Design review of the part shown in the three views and the two pictorial views. Dimensions are in mm from the part's minimum x, y and z. A direction names the side the tool comes from. Give positions to 0.01 mm unless a question says otherwise; leave off trailing zeros. Write each loop counter-clockwise with the first axis right and the second up, starting at its lowest first coordinate (ties: lowest second). Pieces come first, ordered by that corner, then holes. Notation, with made-up numbers: (24.5, -35.5) -> (36.5, -35.5) arc R16 cw to (36.5, -11.5) -> close; hole circle Ø6 at (29, 20). An arc over 180 degrees is marked (long way). Return JSON: item names as keys, results as strings. Group by question number.
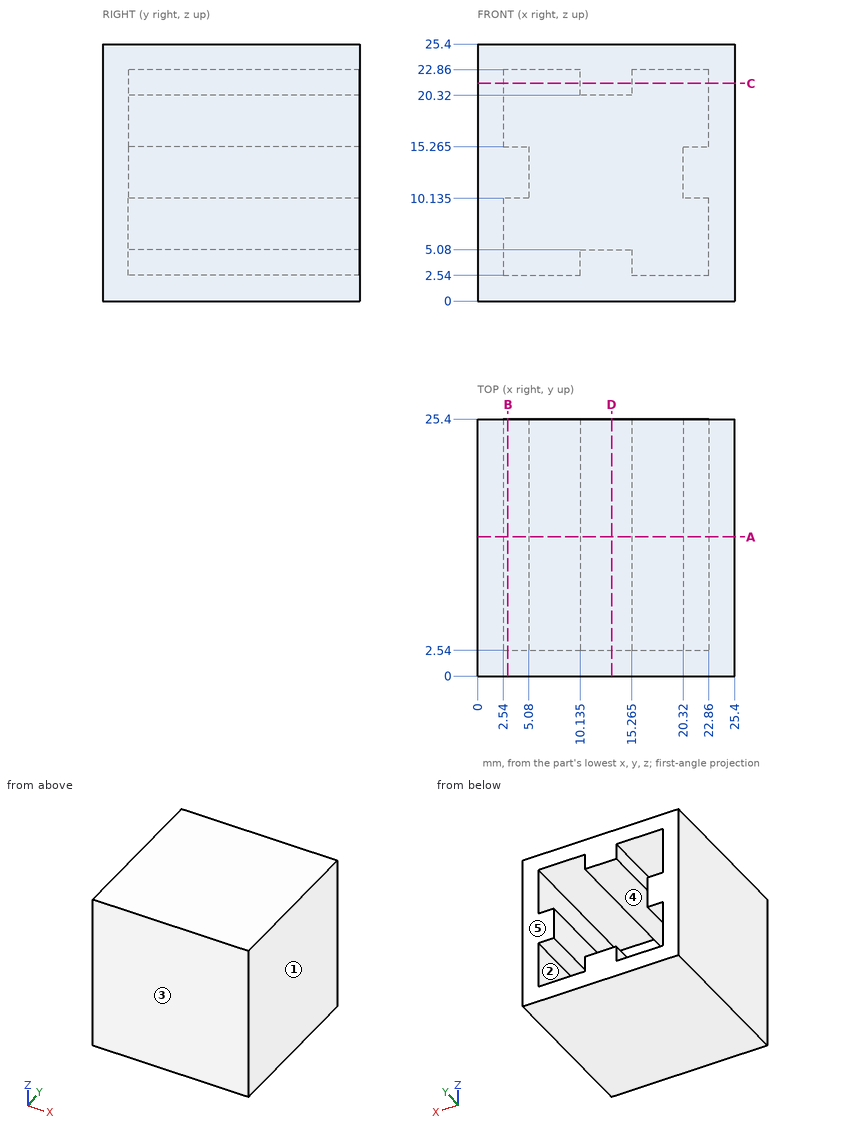
Q1. Take a section at B-B, the plane x = 3. Give the boundary of the cut face in (y, z) (3 decimals).
Q2. Take a section at C-C, the plane z = 21.5. Give the boundary of the cut face in (x, y) (3 decimals).
Q3. Tool access review of the marked faces 4 and 5: name each direction out of +Z, -Z, +X, -X, +Y, -Y from which nothing blocks a thin tool from reaching the whole face with its end or side.
Q4. For L1, parallel to X at y = 8, z = 3.5 (3 decimals); L2, parallel to X at y = 7.75, z = 8, list the stretches that pass through material, from the lowest coordinate up. Write a range as from..to.
Q5. Mouldability with a two-part tool opening along X and no side actions: class the marked faces 1, 2 and 3 as +X half, -X half, draft (parallel to the pull), parting line (faces both ways), or undercut.
Q6. Take a section at A-A, the plane y = 13.75. Give the boundary of the cut face in (x, z) (3 decimals).
Q7. Take a section at D-D, the plane x = 13.25. Give the boundary of the cut face in (y, z).
Final values:
{
 "1": {"outline": "(0, 0) -> (25.4, 0) -> (25.4, 2.54) -> (2.54, 2.54) -> (2.54, 10.135) -> (25.4, 10.135) -> (25.4, 15.265) -> (2.54, 15.265) -> (2.54, 22.86) -> (25.4, 22.86) -> (25.4, 25.4) -> (0, 25.4) -> close"},
 "2": {"outline": "(0, 0) -> (25.4, 0) -> (25.4, 25.4) -> (22.86, 25.4) -> (22.86, 2.54) -> (15.265, 2.54) -> (15.265, 25.4) -> (10.135, 25.4) -> (10.135, 2.54) -> (2.54, 2.54) -> (2.54, 25.4) -> (0, 25.4) -> close"},
 "3": {"face 4": "+Y", "face 5": "+Z, -Z, +X, -X, +Y"},
 "4": {"L1": "x = 0..2.54, 10.135..15.265, 22.86..25.4", "L2": "x = 0..2.54, 22.86..25.4"},
 "5": {"face 1": "+X half", "face 2": "undercut", "face 3": "draft"},
 "6": {"outline": "(0, 0) -> (25.4, 0) -> (25.4, 25.4) -> (0, 25.4) -> close; hole (2.54, 2.54) -> (10.135, 2.54) -> (10.135, 5.08) -> (15.265, 5.08) -> (15.265, 2.54) -> (22.86, 2.54) -> (22.86, 10.135) -> (20.32, 10.135) -> (20.32, 15.265) -> (22.86, 15.265) -> (22.86, 22.86) -> (15.265, 22.86) -> (15.265, 20.32) -> (10.135, 20.32) -> (10.135, 22.86) -> (2.54, 22.86) -> (2.54, 15.265) -> (5.08, 15.265) -> (5.08, 10.135) -> (2.54, 10.135) -> close"},
 "7": {"outline": "(0, 0) -> (25.4, 0) -> (25.4, 5.08) -> (2.54, 5.08) -> (2.54, 20.32) -> (25.4, 20.32) -> (25.4, 25.4) -> (0, 25.4) -> close"}
}
